For this review, use the dimensioned drawing (mm, ordinates from the lowest corner) and the shaded views. Coordinates: 2 decimals unless noted, no trailing zeros. Loops run counter-clockwise (first coordinate to the right, second up) from the corner with the lowest first, then second, coordinate; pieces in that order, holes last. Notation, with made-up numbers: (-35, 24.5) -> (-29, 24.5) arc R36 cw to (-29, 60.5) -> close; hole circle Ø8 at (40.25, -36.75). An arc over 180 degrees is marked (long way). Use one line per item in the form item = value. Start each with the question number.
1. Consider section A-A (x = 395). State the section outline as (y, z) points.
2. Consider section D-D (z = 23). State the section outline as (x, y) points.
3. The part is to be moulded in two halves that separate along Z. For the marked faces 1 and 2, say which applies: released by +Z, released by -Z, zero draft, split by the parting line, or undercut.
4. Wall thickness on line 1 (X direction, y = 177, z = 33); line 2 (Y direction, x = 399, z = 78): over which ranges is each line inside the solid? List them lowest first. Write a range as from..to.
5. Consider section C-C (z = 180). State the section outline as (x, y) points, then the cut area to 3 significant figures.
6. For pin 1 (2 mm diameter, centred on x = 88, z = 231.5, fed in from +Y), flat-tipped, find the tip position at first contact; note if it passes through.
7. Consider section B-B (y = 246.5). State the section outline as (x, z) points, then the cut area to 3 significant figures.
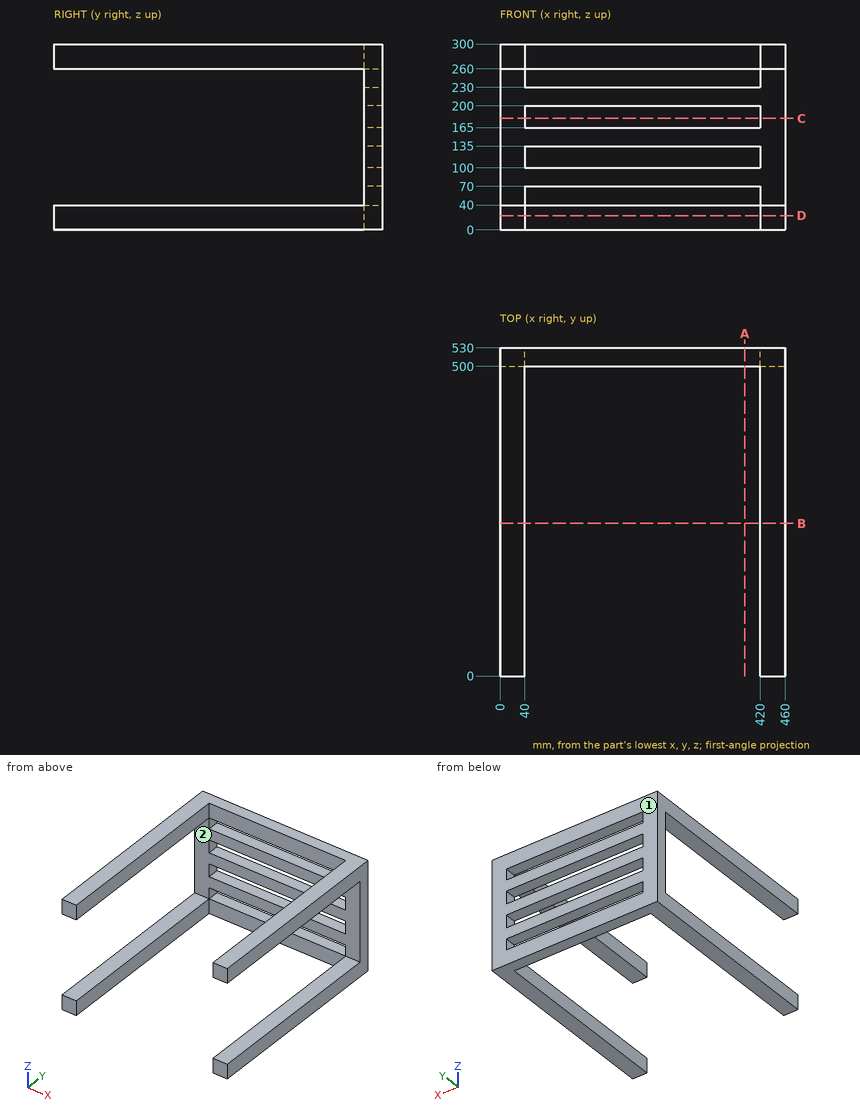
Geometry check:
q1.outline = (500, 0) -> (530, 0) -> (530, 40) -> (500, 40) -> close; (500, 70) -> (530, 70) -> (530, 100) -> (500, 100) -> close; (500, 135) -> (530, 135) -> (530, 165) -> (500, 165) -> close; (500, 200) -> (530, 200) -> (530, 230) -> (500, 230) -> close; (500, 260) -> (530, 260) -> (530, 300) -> (500, 300) -> close
q2.outline = (0, 0) -> (40, 0) -> (40, 500) -> (420, 500) -> (420, 0) -> (460, 0) -> (460, 530) -> (0, 530) -> close
q3.face_1 = zero draft
q3.face_2 = undercut
q4.line_1 = 0..40, 420..460
q4.line_2 = 500..530
q5.outline = (0, 500) -> (40, 500) -> (40, 530) -> (0, 530) -> close; (420, 500) -> (460, 500) -> (460, 530) -> (420, 530) -> close
q5.area = 2,400 mm²
q6.pin_1 = through
q7.outline = (0, 0) -> (40, 0) -> (40, 40) -> (0, 40) -> close; (0, 260) -> (40, 260) -> (40, 300) -> (0, 300) -> close; (420, 0) -> (460, 0) -> (460, 40) -> (420, 40) -> close; (420, 260) -> (460, 260) -> (460, 300) -> (420, 300) -> close
q7.area = 6,400 mm²
